The model under review builds one solid part; all positions refer to its coordinate system, in mm. Give positions to 0.01 mm unless a question says otherwise; leave off trailing zeros. Order: outer loops, then holes, each group sorted by start corner. A loop starts at its lowest first (then second) coordinate and runs counter-clockwise, first axis right, second up. Notation, with made-up numbers: (58, 80) -> (97, 80) arc R17 cw to (97, 96) -> close; hole circle Ø3 at (24, 54.5). An arc over 180 degrees is marked (long way). Answer as a JSON object with one key per item and string values. Group by question number.
from build123d import *

# Parameters (mm, degrees)
BOSS_EXTRUDE1_DEPTH = 6.35
SKETCH2_R           = 3.175
CUT_EXTRUDE1_DEPTH  = 110.433918417
FILLET1_R           = 1


with BuildPart() as part:
    # Sketch1 → Boss-Extrude1 (new body)
    with BuildSketch(Plane(origin=(0, 0, 0), x_dir=(1, 0, 0), z_dir=(0, 1, 0))):
        with BuildLine():
            Line((51.195336702, -25.4), (63.5, -25.4))
            Line((63.5, -25.4), (63.5, -88.9))
            Line((63.5, -88.9), (-63.5, -88.9))
            Line((-63.5, -88.9), (-63.5, -25.4))
            Line((-63.5, -25.4), (-51.195336702, -25.4))
            ThreePointArc((-51.195336702, -25.4), (0, -57.15), (51.195336702, -25.4))
        make_face()
    extrude(amount=BOSS_EXTRUDE1_DEPTH)

    # Sketch2 → Cut-Extrude1 (cut, through all)
    with BuildSketch(Plane(origin=(0, 6.35, 0), x_dir=(-1, 0, 0), z_dir=(0, 1, 0))):
        with Locations(Location((19.05, 69.85, 0), (0, 0, 90))):
            Circle(SKETCH2_R)
        with Locations(Location((-19.05, 69.85, 0), (0, 0, 270))):
            Circle(SKETCH2_R)
        with Locations(Location((-57.15, 69.85, 0), (0, 0, 90))):
            Circle(SKETCH2_R)
        with Locations(Location((57.15, 69.85, 0), (0, 0, 270))):
            Circle(SKETCH2_R)
    extrude(amount=-CUT_EXTRUDE1_DEPTH, mode=Mode.SUBTRACT)

    # Fillet1
    fillet1_edges = [part.edges().sort_by_distance(p)[0] for p in [
        (-63.5, 3.175, 25.4),
        (-51.195336702, 3.175, 25.4),
        (51.195336702, 3.175, 25.4),
        (63.5, 3.175, 25.4),
        (63.5, 3.175, 88.9),
        (-63.5, 3.175, 88.9),
    ]]
    fillet(fillet1_edges, radius=FILLET1_R)


solid = part.part
1. For probe 1 along X at (y, z) = (4.25, 70); probe 2 along Z at (x, y) = (-57.15, 4.5) (3 decimals); probe 3 along X at (y, z) = (5.75, 31.5), list the stretches that pass through material, from the lowest coordinate up. Write a range as [from, to].
2. Take a section at D-D on z = 54.5. Give the boundary of the cut face in (x, y), plus the area to 3 significant figures.
3. Take a section at C-C on x = 57.15. Give the boundary of the cut face in (y, z) (3 decimals), plus the area to 3 significant figures.
4. Take a section at B-B on z = 69.85. Give the boundary of the cut face in (x, y) (3 decimals).
5. Take a section at A-A on y = 2.25. Give the boundary of the cut face in (x, z) (3 decimals), plus the area to 3 significant figures.
6. For pin 1 (5.5 mm diameter, centred on x = 19.05, z = 69.85, fed in from +Y); pin 2 (6 mm diameter, centred on x = -35.5, z = 81.5, fed in from -Y); pin 3 (2 mm diameter, centred on x = 19.5, y = 5.5, fed in from -Z), all flat-tipped, find the tip position at first contact; note any pin that passes through.
7. Draft analysis for pull direction X (two halves, no side actions). For faces 1 (the cylindrical face through (-18.91, 3.22, 66.68)), 2 (the flat face through (-63.5, 3, 58)), 3 (the flat face through (63.5, 3, 57)), 4 (the flat face through (1, 3, 88.9)), state which applies: pulls with the +X half, pulls with the -X half, needs draft (parallel to the pull), parting line crosses it, or undercut.
Checks:
{
 "1": {"probe 1": "x = [-63.5, -60.32], [-53.98, -22.22], [-15.88, 15.88], [22.22, 53.98], [60.32, 63.5]", "probe 2": "z = [25.4, 66.675], [73.025, 88.9]", "probe 3": "x = [-63.5, -47.69], [47.69, 63.5]"},
 "2": {"outline": "(-63.5, 0) -> (-17.2, 0) -> (-17.2, 6.35) -> (-63.5, 6.35) -> close; (17.2, 0) -> (63.5, 0) -> (63.5, 6.35) -> (17.2, 6.35) -> close", "area": "588 mm2"},
 "3": {"outline": "(0, 25.4) -> (6.35, 25.4) -> (6.35, 66.675) -> (0, 66.675) -> close; (0, 73.025) -> (6.35, 73.025) -> (6.35, 88.9) -> (0, 88.9) -> close", "area": "363 mm2"},
 "4": {"outline": "(-63.5, 0) -> (-60.325, 0) -> (-60.325, 6.35) -> (-63.5, 6.35) -> close; (-53.975, 0) -> (-22.225, 0) -> (-22.225, 6.35) -> (-53.975, 6.35) -> close; (-15.875, 0) -> (15.875, 0) -> (15.875, 6.35) -> (-15.875, 6.35) -> close; (22.225, 0) -> (53.975, 0) -> (53.975, 6.35) -> (22.225, 6.35) -> close; (60.325, 0) -> (63.5, 0) -> (63.5, 6.35) -> (60.325, 6.35) -> close"},
 "5": {"outline": "(-63.5, 26.4) arc R1 ccw to (-62.5, 25.4) -> (-51.812, 25.4) arc R1 ccw to (-50.921, 25.946) arc R57.15 cw to (50.921, 25.946) arc R1 ccw to (51.812, 25.4) -> (62.5, 25.4) arc R1 ccw to (63.5, 26.4) -> (63.5, 87.9) arc R1 ccw to (62.5, 88.9) -> (-62.5, 88.9) arc R1 ccw to (-63.5, 87.9) -> close; hole circle Ø6.35 at (-57.15, 69.85); hole circle Ø6.35 at (-19.05, 69.85); hole circle Ø6.35 at (19.05, 69.85); hole circle Ø6.35 at (57.15, 69.85)", "area": "5,610 mm2"},
 "6": {"pin 1": "passes through", "pin 2": "stops at y = 0", "pin 3": "stops at z = 53.35"},
 "7": {"face 1": "undercut", "face 2": "pulls with the -X half", "face 3": "pulls with the +X half", "face 4": "needs draft"}
}
